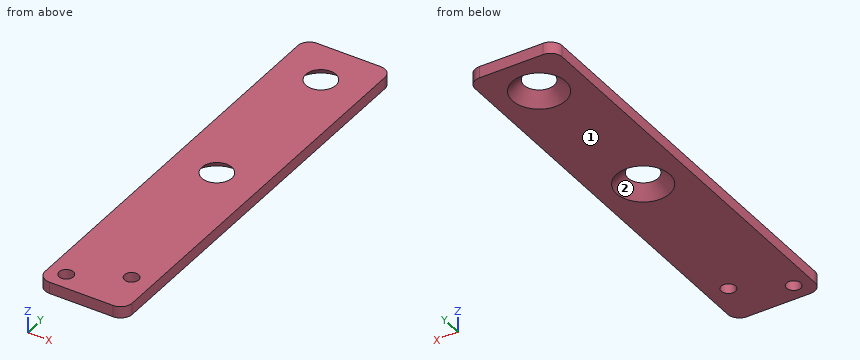
Solid Edge part; units mm, degrees
sketch "Sketch1" plane through (0, 0, 0) normal (0, 0, 1) x (1, 0, 0)
  line L0 (15, -72) -> (0, -72)
  line L1 (0, -72) -> (0, 0)
  line L2 (0, 0) -> (15, 0)
  line L3 (15, 0) -> (15, -72)
extrude "Protrusion1" add sketch "Sketch1" along normal blind 2
hole "Bohrung_1" at (3, -69, 2) direction (0, 0, -1) diameter 2.459 end through all
hole "Hole1" at (11.388, -64.54, 2) direction (0, 0, -1) diameter 2.459 end through all
fillet "Verrundung_1" radius 2 4 edges at (15, 0, 1) (0, 0, 1) (15, -72, 1) (0, -72, 1)
hole "Bohrung_5" at (7.5, -35.5, 0) direction (0, 0, 1) diameter 4.3 end through all countersink diameter 9.18 countersink angle 90
hole "Hole2" at (7.5, -7.5, 0) direction (0, 0, 1) diameter 4.3 end through all countersink diameter 9.18 countersink angle 90
CAD build for the part. Positions are in the model's coordinates, mm. Face numbers are marked on the shaded views. Round coordinates to 2 decimals unless told otherwise and drop trailing zeros. Order: outer loops, then holes, each group sorted by start corner. A loop starts at its lowest first (then second) coordinate and runs counter-clockwise, first axis right, second up. Notation, with made-up numbers: (-32.75, -37.5) - (-9.75, -37.5) arc R27 ccw to (-9.75, -13.5) - close; hole circle Ø11 at (45, 1.5). An arc over 180 degrees is marked (long way). Use CSV: the item, a comma, the result in double quotes. Start each with the question number.
1) Pin check, flat tips, straight feed: pin 1 Ø6 at (x, y) = (4, -36) entering from -Z; pin 2 Ø2 at (x, y) = (3, -69) entering from -Z. Stop position of each tip, or through.
2) Saw through at D-D (y = -69). List the corners of the cut face in (x, z), and give its area (3 significant figures).
3) Saw through at C-C (z = 0.6). List the corners of the cut face in (x, y), and give its area (3 significant figures).
4) Two-plate mould, pull along X, no slides. Class the marked faces 1 and 2: pulls with the +X half, pulls with the -X half, needs draft (parallel to the pull), parting line crosses it, or undercut.
5) Wall check: L1, parallel to X at y = -64.5, z = 0.95; L2, parallel to Y at x = 4, z = 0.45; L3, parallel to Y at x = 3, z = 1.25. Give the ranges that are in metal, low to high. Write a range as [from, to].
6) Saw through at A-A (y = -35.5). List the corners of the cut face in (x, z), and give its area (3 significant figures).
7) Saw through at B-B (x = 7.5). List the corners of the cut face in (y, z), and give its area (3 significant figures).
Values follow:
1,pin 1,"stops at z = 0"
1,pin 2,"passes through"
2,outline,"(0, 0) - (1.77, 0) - (1.77, 2) - (0, 2) - close; (4.23, 0) - (15, 0) - (15, 2) - (4.23, 2) - close"
2,area,"25.1 mm2"
3,outline,"(0, -70) arc R2 ccw to (2, -72) - (13, -72) arc R2 ccw to (15, -70) - (15, -2) arc R2 ccw to (13, 0) - (2, 0) arc R2 ccw to (0, -2) - close; hole circle Ø2.46 at (3, -69); hole circle Ø7.98 at (7.5, -35.5); hole circle Ø7.98 at (7.5, -7.5); hole circle Ø2.46 at (11.39, -64.54)"
3,area,"967 mm2"
4,face 1,"needs draft"
4,face 2,"undercut"
5,L1,"x = [0, 10.16], [12.62, 15]"
5,L2,"y = [-72, -69.72], [-68.28, -37.71], [-33.29, -9.71], [-5.29, 0]"
5,L3,"y = [-72, -70.23], [-67.77, 0]"
6,outline,"(0, 0) - (2.91, 0) - (4.91, 2) - (0, 2) - close; (10.09, 2) - (12.09, 0) - (15, 0) - (15, 2) - close"
6,area,"15.6 mm2"
7,outline,"(-72, 0) - (-40.09, 0) - (-38.09, 2) - (-72, 2) - close; (-32.91, 2) - (-30.91, 0) - (-12.09, 0) - (-10.09, 2) - close; (-4.91, 2) - (-2.91, 0) - (0, 0) - (0, 2) - close"
7,area,"115 mm2"
